Design review of the part shown in the three views and the two pictorial views. Dimensions are in mm from the part's minimum x, y and z. A direction names the side the tool comes from. Give positions to 0.01 mm unless a question says otherwise; leave off trailing zeros. Loops run counter-clockwise (first coordinate to the right, second up) from the corner with the lowest first, then second, coordinate; pieces in that order, holes last. Notation, with made-up numbers: (-36.5, 44.5) -> (-3.5, 44.5) arc R24 cw to (-3.5, 71.5) -> close; hole circle Ø6 at (78.5, 56). An arc over 180 degrees is marked (long way). One line per question, with ' | ' between items. Start each with the question number.
(1) Tool access review of the marked faces 1 and 2: name each direction out of +Z, -Z, +X, -X, +Y, -Y from which nothing blocks a thin tool from reaching the whole face with its end or side.
(2) Consider section B-B (x = 8.5). Write out the cut boundary in (y, z).
(3) Consider section D-D (z = 70). Write out the cut boundary in (x, y).
(4) Consider section A-A (y = 2.7). Write out the cut boundary in (x, z), and give its area (3 significant figures).
(5) Insertion check: P1, Ø0.6, axis at x = 12, y = 2.5, coming from the -Z side; P2, Ø6, axis at x = 5.5, z = 88.5, coming from the +Y side. Each pin has a flat end and moves straight along its axis. Give the tip position at first contact, or say it passes through.
(6) Consider section C-C (z = 95.7). Write out the cut boundary in (x, y).
(7) Wall thickness on probe 1 along Z at (x, y) = (5, 2.05); probe 2 along X at (y, z) = (1.95, 95.7); probe 3 along Z at (x, y) = (16.75, 3.8): over which ranges is each line inside the solid? List them lowest first.
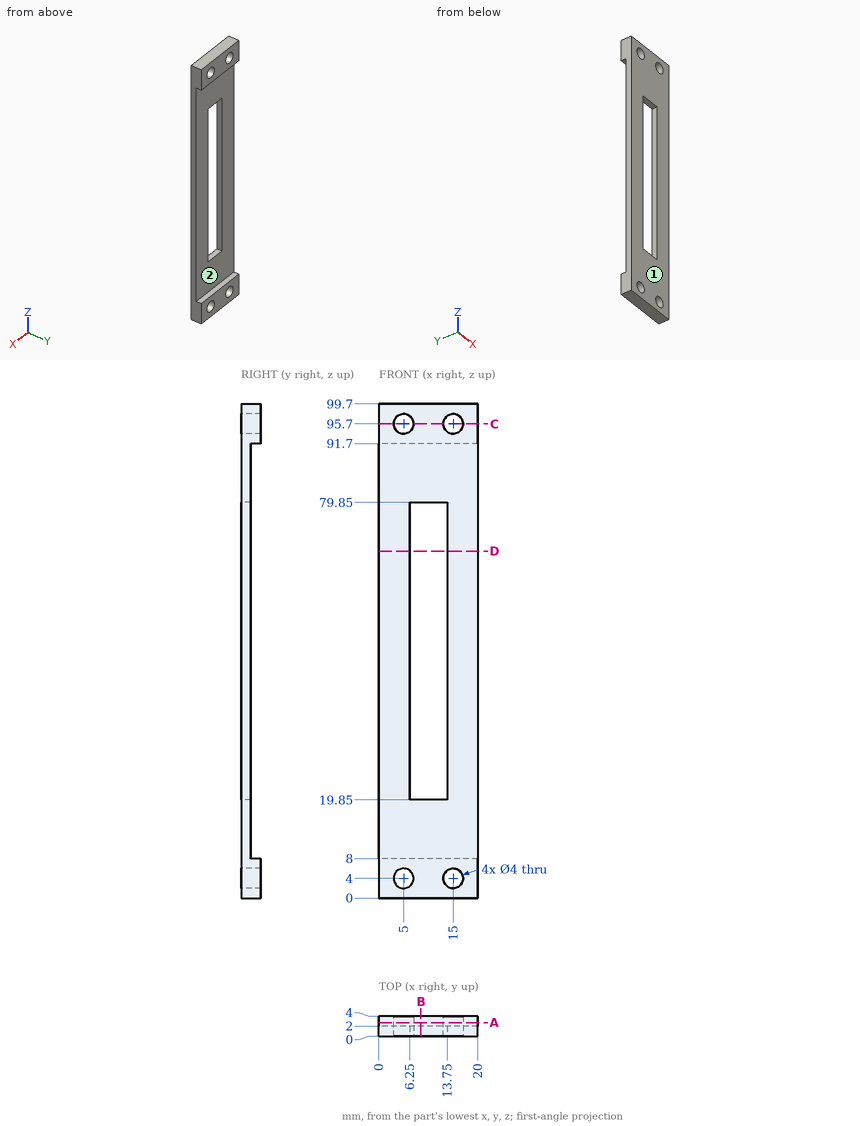
A:
1) face 1: +Z, -Z, +X, -X, -Y | face 2: +X, -X, +Y
2) outline: (0, 0) -> (4, 0) -> (4, 8) -> (2, 8) -> (2, 19.85) -> (0, 19.85) -> close; (0, 79.85) -> (2, 79.85) -> (2, 91.7) -> (4, 91.7) -> (4, 99.7) -> (0, 99.7) -> close
3) outline: (0, 0) -> (6.25, 0) -> (6.25, 2) -> (0, 2) -> close; (13.75, 0) -> (20, 0) -> (20, 2) -> (13.75, 2) -> close
4) outline: (0, 0) -> (20, 0) -> (20, 8) -> (0, 8) -> close; (0, 91.7) -> (20, 91.7) -> (20, 99.7) -> (0, 99.7) -> close; hole circle Ø4 at (5, 4); hole circle Ø4 at (5, 95.7); hole circle Ø4 at (15, 4); hole circle Ø4 at (15, 95.7) | area: 270 mm^2
5) P1: stops at z = 0 | P2: stops at y = 2
6) outline: (0, 0) -> (3, 0) -> (3, 4) -> (0, 4) -> close; (7, 0) -> (13, 0) -> (13, 4) -> (7, 4) -> close; (17, 0) -> (20, 0) -> (20, 4) -> (17, 4) -> close
7) probe 1: z = 0 to 2, 6 to 8, 91.7 to 93.7, 97.7 to 99.7 | probe 2: x = 0 to 3, 7 to 13, 17 to 20 | probe 3: z = 0 to 3.03, 4.97 to 8, 91.7 to 94.73, 96.67 to 99.7
